Part model, mm, in its own coordinate system. Face numbers are marked on the shaded views. A direction names the side the tool comes from. Coordinates: 2 decimals unless noted, no trailing zeros. Write each loop counter-clockwise with the first axis right and the second up, starting at its lowest first coordinate (ties: lowest second). Pieces come first, ordered by that corner, then holes. Notation, with made-up numbers: (34, 35.25) - (79, 35.25) arc R24 cw to (79, 45.25) - close; hole circle Ø6 at (-32, 49.25). An arc over 180 degrees is marked (long way). Use a Markdown table: item, result.
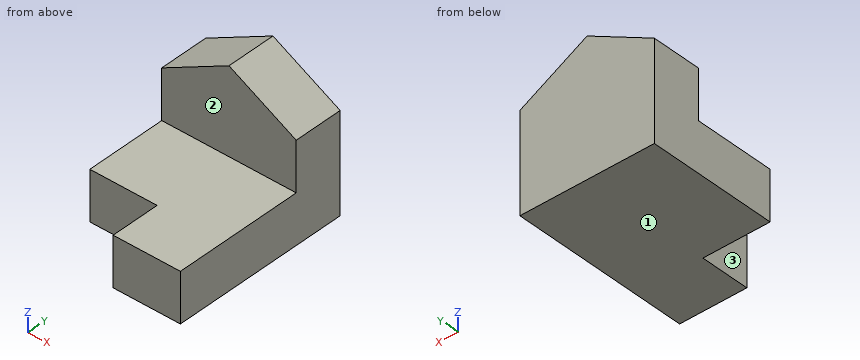
```python
from build123d import *

# Parameters (mm, degrees)
F1_DEPTH  = 30
F2_W      = 11
F2_H      = 15
F3_DEPTH  = 11
F4_W      = 15
F4_H      = 8
F5_DEPTH  = 11
F6_ANGLE  = -90
F8_DEPTH  = 11
F10_DEPTH = 11


with BuildPart() as f1:
    # F0 (on Front) → F1 (new body)
    with BuildSketch(Plane.XZ):
        Polygon((0, 30), (0, 0), (40, 0), (40, 11), (11, 11), (11, 30), align=None)
    extrude(amount=F1_DEPTH)

    # F2 (on face) → F3 (cut, through all)
    with BuildSketch(Plane.XY.offset(11)):
        with Locations((34.5, -22.5)):
            Rectangle(F2_W, F2_H)
    extrude(amount=-F3_DEPTH, mode=Mode.SUBTRACT)

    # F4 (on face) → F5 (cut, through all)
    with BuildSketch(Plane.YZ.offset(11)):
        with Locations((-22.5, 26)):
            Rectangle(F4_W, F4_H)
    extrude(amount=-F5_DEPTH, mode=Mode.SUBTRACT)


with BuildPart() as f1_1:
    # F6: moved
    add(f1.part.rotate(Axis((0, 0, 15), (0, 0, 1)), F6_ANGLE))

    # F7 (on face) → F8 (join, through all)
    with BuildSketch(Plane.XZ.offset(11)):
        Polygon((-15, 22), (-15, 30), (-30, 22), align=None)
    extrude(amount=-F8_DEPTH)

    # F9 (on face) → F10 (cut, through all)
    with BuildSketch(Plane.XZ.offset(11)):
        Polygon((0, 30), (-15, 30), (0, 22), align=None)
    extrude(amount=-F10_DEPTH, mode=Mode.SUBTRACT)


solid = f1_1.part
```
Item 1: Band-saw the part on C-C, the plane y = -25. Give the cut face in (x, z), then the cut area to 3 significant figures.
From the geometry:
| item | result |
|---|---|
| outline | (-30, 0) - (0, 0) - (0, 11) - (-30, 11) - close |
| area | 330 mm^2 |
Item 2: Drop flat-ended pins along their axis: P1, Ø5.5, axis at y = -37, z = 7.5, coming from the -X side; P2, Ø8.5, axis at x = -18.5, y = -21, coming from the +Z side; P3, Ø6, axis at x = -15.5, z = 17, coming from the -Y side. Give the stop position or say it passes through.
From the geometry:
| item | result |
|---|---|
| P1 | x = -15 |
| P2 | z = 11 |
| P3 | y = -11 |
Item 3: Which spindle directions (+Z, -Z, +X, -X, +Y, -Y) get a long thin tool onto all of the face, cutting with end or side? Do the marked faces 1, 2 and 3. Say none if no direction does.
From the geometry:
| item | result |
|---|---|
| face 1 | -Z, +X, -X, +Y, -Y |
| face 2 | +Z, +X, -X, -Y |
| face 3 | +Z, -Z, -X, -Y |
Item 4: Band-saw the part on A-A, the plane z = 5.5. Give the cut face in (x, y).
From the geometry:
| item | result |
|---|---|
| outline | (-30, -29) - (-15, -29) - (-15, -40) - (0, -40) - (0, 0) - (-30, 0) - close |
Item 5: Band-saw the part on B-B, the plane x = -21. Give the cut face in (y, z), then the cut area to 3 significant figures.
From the geometry:
| item | result |
|---|---|
| outline | (-29, 0) - (0, 0) - (0, 26.8) - (-11, 26.8) - (-11, 11) - (-29, 11) - close |
| area | 493 mm^2 |
Item 6: Drill centre lines: probe 1 along Z at (x, y) = (-13.5, -25.5); probe 2 along Y at (x, z) = (-16.5, 26.5); probe 3 along Y at (x, z) = (-21.5, 5.5). Where is each one in solid material? Low to high.
From the geometry:
| item | result |
|---|---|
| probe 1 | 0 to 11 |
| probe 2 | -11 to 0 |
| probe 3 | -29 to 0 |
Item 7: Band-saw the part on D-D, the plane z = 20.5. Give the cut face in (x, y).
From the geometry:
| item | result |
|---|---|
| outline | (-30, -11) - (0, -11) - (0, 0) - (-30, 0) - close |
